```python
from build123d import *

# Parameters (mm, degrees)
SKETCH1_W           = 31
SKETCH1_H           = 45.4
BOSS_EXTRUDE1_DEPTH = 13
SKETCH2_W           = 27
SKETCH2_H           = 11
CUT_EXTRUDE1_DEPTH  = 57.490353159
SKETCH3_R           = 1.6
CUT_EXTRUDE2_DEPTH  = 10
SKETCH4_W           = 15
SKETCH4_H           = 13
BOSS_EXTRUDE2_DEPTH = 15
SKETCH5_R           = 1.75
CUT_EXTRUDE3_DEPTH  = 20
FILLET1_R           = 5
BOSS_EXTRUDE3_DEPTH = 15
CHAMFER1_SIZE       = 5
CUT_EXTRUDE4_DEPTH  = 4


with BuildPart() as part:
    # Sketch1 → Boss-Extrude1 (new body)
    with BuildSketch(Plane(origin=(0, 0, 0), x_dir=(1, 0, 0), z_dir=(0, 1, 0))):
        with Locations((15.5, 22.7)):
            Rectangle(SKETCH1_W, SKETCH1_H)
    extrude(amount=BOSS_EXTRUDE1_DEPTH)

    # Sketch2 → Cut-Extrude1 (cut, through all)
    with BuildSketch(Plane.XY):
        with Locations((15.5, 5.5)):
            Rectangle(SKETCH2_W, SKETCH2_H)
    extrude(amount=-CUT_EXTRUDE1_DEPTH, mode=Mode.SUBTRACT)

    # Sketch3 → Cut-Extrude2 (cut)
    with BuildSketch(Plane(origin=(0, 13, 0), x_dir=(1, 0, 0), z_dir=(0, 1, 0))):
        with Locations(Location((5.5, 32.7, 0), (0, 0, 270))):
            Circle(SKETCH3_R)
        with Locations(Location((25.5, 32.7, 0), (0, 0, 270))):
            Circle(SKETCH3_R)
        with Locations(Location((25.5, 12.7, 0), (0, 0, 270))):
            Circle(SKETCH3_R)
        with Locations(Location((5.5, 12.7, 0), (0, 0, 270))):
            Circle(SKETCH3_R)
    extrude(amount=-CUT_EXTRUDE2_DEPTH, mode=Mode.SUBTRACT)

    # Sketch4 → Boss-Extrude2 (add)
    with BuildSketch(Plane.ZY):
        with Locations((-7.5, 6.5)):
            Rectangle(SKETCH4_W, SKETCH4_H)
    extrude(amount=BOSS_EXTRUDE2_DEPTH)

    # Sketch5 → Cut-Extrude3 (cut)
    with BuildSketch(Plane(origin=(0, 13, 0), x_dir=(1, 0, 0), z_dir=(0, 1, 0))):
        with Locations(Location((-10, 5, 0), (0, 0, 270))):
            Circle(SKETCH5_R)
    extrude(amount=-CUT_EXTRUDE3_DEPTH, mode=Mode.SUBTRACT)

    # Fillet1
    fillet1_edges = [part.edges().sort_by_distance(p)[0] for p in [
        (-15, 6.5, -15),
        (-15, 6.5, 0),
    ]]
    fillet(fillet1_edges, radius=FILLET1_R)

    # Sketch6 → Boss-Extrude3 (add)
    with BuildSketch(Plane(origin=(31, 0, 0), x_dir=(0, 0, -1), z_dir=(1, 0, 0))):
        Polygon((5, 0), (10, 0), (10, 5.8), (30, 5.8), (30, 0), (35, 0), (35, 13), (5, 13), align=None)
    extrude(amount=BOSS_EXTRUDE3_DEPTH)

    # Chamfer1
    chamfer1_edges = [part.edges().sort_by_distance(p)[0] for p in [
        (38.5, 0, -5),
        (38.5, 0, -35),
    ]]
    chamfer(chamfer1_edges, length=CHAMFER1_SIZE - 0.0001)  # a hair under: the kernel refuses the full size

    # Sketch7 → Cut-Extrude4 (cut)
    with BuildSketch(Plane(origin=(43, 0, 0), x_dir=(0, 0, -1), z_dir=(1, 0, 0))):
        Polygon((5, 8), (15, 13), (5, 13), align=None)
        Polygon((35, 8), (25, 13), (35, 13), align=None)
    extrude(amount=-CUT_EXTRUDE4_DEPTH, mode=Mode.SUBTRACT)


solid = part.part
```
Source: CAD feature listing. Evaluate the final solid. Frame: model axes, mm. A direction names the side the tool comes from. Round coordinates to 2 decimals unless told otherwise and drop trailing zeros. Loops run counter-clockwise (first coordinate to the right, second up) from the corner with the lowest first, then second, coordinate; pieces in that order, holes last.
1. Contact query for flat-ended pins moving along their axis: pin 1 (1 mm diameter, centred on x = 3.5, y = 5.5, fed in from +Z); pin 2 (4 mm diameter, centred on x = 25.5, z = -12.7, fed in from -Y); pin 3 (2.5 mm diameter, centred on y = 10, z = -30.5, fed in from -X); pin 4 (5 mm diameter, centred on x = -3.5, y = 6, fed in from -Z). Output: stop coordinate, or through.
2. Access query for faces 1 (the flat face through (39, 11, -9)), 2 (the flat face through (15, 11, -22)), 3 (the flat face through (38, 3, -30)). Directions: +Z, -Z, +X, -X, +Y, -Y. A direction counts if a zero-diameter tool reaches every point of the face in a straight line with its end or side. Return the directions, or none.
3. Section query B-B on y = 1. Output: boundary loops of the cut face in (x, z).
4. Section query C-C on z = -16. Output: boundary loops of the cut face in (x, y), and give its area (3 significant figures).
5. Mould query, pull axis Z, two halves, no side actions, for faces 4 (the flat face through (1.7, 6.4, 0)), 5 (the flat face through (29, 5, -22)), 6 (the flat face through (38, 3, -10)). Classes: released by +Z, released by -Z, zero draft, split by the parting line, or undercut.
6. Ray query, L1, parallel to X at y = 11.4, z = -32.7; L2, parallel to X at y = 4.75, z = -21; L3, parallel to X at y = 10, z = -30. Return the intervals inside material, ascending.
7. Section query A-A on x = 25.5. Output: boundary loops of the cut face in (y, z).
Answers below:
1. pin 1: passes through
1. pin 2: stops at y = 11
1. pin 3: stops at x = 0
1. pin 4: stops at z = -15
2. face 1: +Z, +Y
2. face 2: +Z, -Z, -Y
2. face 3: +X, -Y
3. outline: (-15, -10) arc R5 ccw to (-10, -15) - (0, -15) - (0, -45.4) - (2, -45.4) - (2, 0) - (-10, 0) arc R5 ccw to (-15, -5) - close; (29, -45.4) - (31, -45.4) - (31, -31) - (46, -31) - (46, -30) - (31, -30) - (31, -10) - (46, -10) - (46, -9) - (31, -9) - (31, 0) - (29, 0) - close; hole circle Ø3.5 at (-10, -5)
4. outline: (0, 0) - (2, 0) - (2, 11) - (29, 11) - (29, 0) - (31, 0) - (31, 5.8) - (46, 5.8) - (46, 13) - (0, 13) - close
4. area: 214 mm2
5. face 4: released by +Z
5. face 5: zero draft
5. face 6: undercut
6. L1: x = 0 to 3.9, 7.1 to 23.9, 27.1 to 39, 43 to 46
6. L2: x = 0 to 2, 29 to 31
6. L3: x = 0 to 2, 29 to 46
7. outline: (11, -45.4) - (13, -45.4) - (13, -34.3) - (11, -34.3) - close; (11, -31.1) - (13, -31.1) - (13, -14.3) - (11, -14.3) - close; (11, -11.1) - (13, -11.1) - (13, 0) - (11, 0) - close
